Can you work these out from the model? Positions are in its coordinate system, mm. Face numbers are marked on the shaded views. Coordinates: 2 decimals unless noted, no trailing zeros. Loops run counter-clockwise (first coordinate to the right, second up) from the corner with the lowest first, then second, coordinate; pieces in that order, holes last. Notation, with made-up numbers: (16.5, -17.75) - (51.5, -17.75) arc R22 cw to (51.5, 19.25) - close; hole circle Ø1 at (17, 66). An arc over 180 degrees is marked (long way). Put each result on its own line as item: value. Start each with the question number.
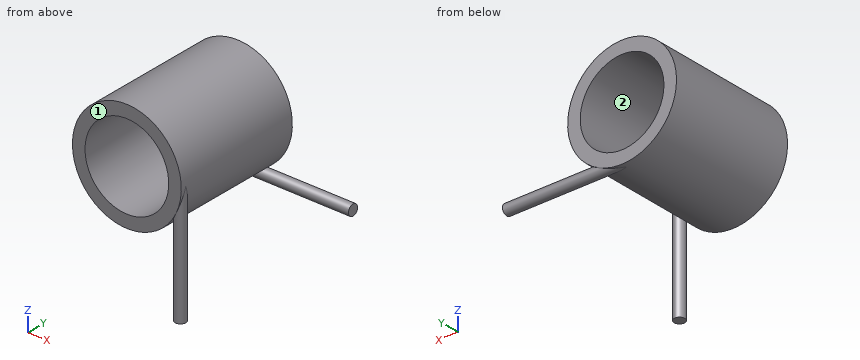
Autodesk Inventor part; units mm, degrees
ref_plane "YZ Plane" through (0, 0, 0) normal (1, 0, 0) x (0, 1, 0)
ref_plane "XZ Plane" through (0, 0, 0) normal (0, 1, 0) x (-1, 0, 0)
ref_plane "XY Plane" through (0, 0, 0) normal (0, 0, 1) x (1, 0, 0)
sketch "Sketch1" plane through (0, 0, 0) normal (0, 1, 0) x (-1, 0, 0)
  circle A0 centre (0, 0) radius 4.55
  circle A1 centre (0, 0) radius 3.5
  dimension "d0" = 9.1
  dimension "d1" = 7
extrude "Extrusion1" add sketch "Sketch1" along normal blind 11
sketch "Sketch2" plane through (0, 0, 0) normal (0, 0, 1) x (1, 0, 0)
  line L0 (4.55, 11) -> (-4.55, 11)
  line L1 (4.55, 0) -> (-4.55, 0)
  line L2 (4.55, 0) -> (-4.55, 0)
  line L3 (4.55, 0) -> (4.55, 11)
  line L4 (-4.55, 0) -> (-4.55, 11)
  circle A0 centre (4.1, 0.45) radius 0.45
  point P0 (0, 0)
  dimension "d11" = 0.9
extrude "Extrusion2" add sketch "Sketch2" against normal blind 10 contours A0
sketch "Sketch3" plane through (0, 0, 0) normal (1, 0, 0) x (0, 1, 0)
  line L0 (0, -4.55) -> (0, 4.55)
  line L1 (11, -4.55) -> (11, 4.55)
  line L2 (11, -4.55) -> (11, 4.55)
  line L3 (0, 4.55) -> (11, 4.55)
  line L4 (0, -4.55) -> (11, -4.55)
  circle A0 centre (10.55, -4.1) radius 0.45
  point P0 (0, 0)
  point P1 (0, -1.9729)
  point P2 (0.45, 0)
  dimension "d12" = 0.9
extrude "Extrusion3" add sketch "Sketch3" along normal blind 10 contours A0
properties part number "Torsion_spring"
Q1. Will these pins go through, and if not, where does the flat tip stop? pin 1 (6 mm diameter, centred on x = 5, y = 8, fed in from +Z); pin 2 (2 mm diameter, centred on y = 8, z = 1.5, fed in from +X); pin 3 (2 mm diameter, centred on y = 7.5, z = -4.5, fed in from +X).
Q2. I want a section at C-C on x = -2.75. List the corners of the cut face in (y, z) for me, and give its area (3 significant figures).
Q3. I want a section at B-B on y = 7. List the corners of the cut face in (x, z) for me.
Q4. We'd pull the mould along Z, two halves only. Please class the marked faces 1 and 2: released by +Z, released by -Z, zero draft, split by the parting line, or undercut.
Q5. I want a section at D-D on x = 8. List the corners of the cut face in (y, z) for me, and give its area (3 significant figures).
Q6. I want a section at A-A on z = -1. List the corners of the cut face in (x, y) for me.
Q7. Please list where these lines run through material, in increasing order: line 1 along Z through (x, y) = (0, 5.25); line 2 along Z through (x, y) = (-3, 5); line 3 along X through (y, z) = (5, -2.5). Write a range as [from, to].
Calculated:
1. pin 1: z = 4.09
1. pin 2: x = 4.52
1. pin 3: x = 2.91
2. outline: (0, -3.62) - (11, -3.62) - (11, -2.17) - (0, -2.17) - close; (0, 2.17) - (11, 2.17) - (11, 3.62) - (0, 3.62) - close
2. area: 32.1 mm2
3. outline: circle Ø9.1 at (0, 0); hole circle Ø7 at (0, 0)
4. face 1: zero draft
4. face 2: undercut
5. outline: circle Ø0.9 at (10.55, -4.1)
5. area: 0.636 mm2
6. outline: (-4.44, 0) - (-3.35, 0) - (-3.35, 11) - (-4.44, 11) - close; (3.35, 0) - (4.44, 0) - (4.44, 0.15) arc R0.45 ccw to (4.44, 0.75) - (4.44, 11) - (3.35, 11) - close
7. line 1: [-4.55, -3.5], [3.5, 4.55]
7. line 2: [-3.42, -1.8], [1.8, 3.42]
7. line 3: [-3.8, -2.45], [2.45, 3.8]
